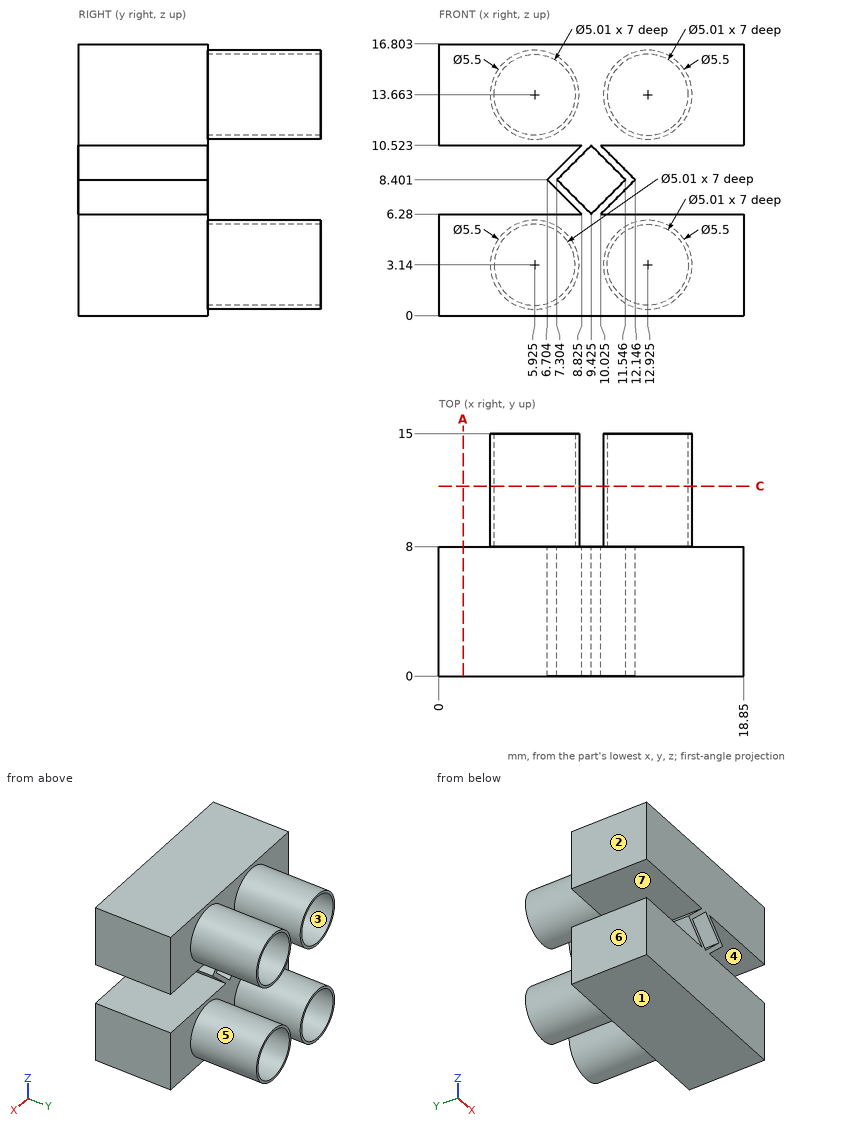
Source: three-view drawing plus pictorial views. Frame: mm from the lowest corner of the part. A direction names the side the tool comes from. Coordinates: 2 decimals unless noted, no trailing zeros. Write each loop counter-clockwise with the first axis right and the second up, starting at its lowest first coordinate (ties: lowest second). Pieces come first, ordered by that corner, then holes. Notation, with made-up numbers: (-7.5, -27.75) -> (17.5, -27.75) arc R22 cw to (17.5, 10.25) -> close; hole circle Ø1 at (25, 40.25). An arc over 180 degrees is marked (long way). Answer as a JSON object with one key per item and string values.
1. Section C-C on y = 11.75. Count the separate pieces of the cut face and the enclosed holes in it.
Result set:
{"separate pieces": "4", "enclosed holes": "4"}
2. Mould query, pull axis Z, two halves, no side actions, for the marked faces 1, 2 and 3. Classes: released by +Z, released by -Z, zero draft, split by the parting line, or undercut.
Result set:
{"face 1": "released by -Z", "face 2": "zero draft", "face 3": "undercut"}
3. First-contact query: P1, Ø1, axis at x = 6.5, y = 11, coming from the +Z side; P2, Ø3, axis at x = 12.92, z = 13.66, coming from the +Y side. Flat tips, straight axial feed; report the tip coordinate or a pass-through.
Result set:
{"P1": "stops at z = 16.41", "P2": "stops at y = 8"}
4. Section A-A on x = 1.5. Return the cut outline in (y, z).
Result set:
{"outline": "(0, 0) -> (8, 0) -> (8, 6.28) -> (0, 6.28) -> close; (0, 10.52) -> (8, 10.52) -> (8, 16.8) -> (0, 16.8) -> close"}
5. Access query for the marked faces 4, 5, 6 and 7. Directions: +Z, -Z, +X, -X, +Y, -Y. A direction counts if a zero-diameter tool reaches every point of the face in a straight line with its end or side. Return the directions, or none.
Result set:
{"face 4": "+X, +Y, -Y", "face 5": "+Y", "face 6": "+Z, -Z, -X, +Y, -Y", "face 7": "-X, +Y, -Y"}
6. Material intervals for line 1 (Z direction, x = 12.75, y = 6.25); line 2 (Z direction, x = 11.25, y = 9.25) (1 decimal); line 3 (X direction, y = 11, z = 15), sorted ascending. Write a range as from..to.
Result set:
{"line 1": "z = 0..6.28, 10.52..16.8", "line 2": "z = 1..1.3, 5..5.3, 11.5..11.8, 15.5..15.8", "line 3": "x = 3.52..3.81, 8.04..8.33, 10.52..10.81, 15.04..15.33"}
